The listing builds one solid part. Answer for the finished solid, in the listing's coordinates (mm). A direction names the side the tool comes from. Coordinates: 2 decimals unless noted, no trailing zeros. Order: outer loops, then holes, each group sorted by start corner. A loop starts at its lowest first (then second) coordinate and runs counter-clockwise, first axis right, second up. Notation, with made-up numbers: (57.5, 57) - (86.5, 57) arc R9 cw to (86.5, 72) - close; hole circle Ø1 at (80, 23.5). An arc over 180 degrees is marked (long way). Use one line per item in the form item = value. Start each with the question number.
Item 1: Section B-B, the plane z = 12.54 is taken. Write down the section's boundary in (x, y), and give its area (3 significant figures).
Item 2: The mould has two halves that part along Z. Classify faces 1 (the cylindrical face through (66.99, -12.727, 2.504)), 2 (the cylindrical face through (77.591, -2.576, 11.487)), 3 (the flat face through (83.4, -12.64, 12.44)): released by +Z, released by -Z, zero draft, split by the parting line, or undercut.
Item 3: Section D-D, the plane x = 42.5 is taken. Write down the section's boundary in (y, z), and give its area (3 significant figures).
Item 4: A tool of negligible diameter and unlimited length cuts with its end or side. For faces 4 (the flat face through (25.94, -12.64, 12.44)), 5 (the flat face through (71, -12, 5.08)), from which of +Z, -Z, +X, -X, +Y, -Y can it reach the whole face along a straight path? Write none if from no direction.
Item 5: Section A-A, the plane y = -10 is taken. Write down the section's boundary in (x, z).
Item 6: Consider line 1 along X through (y, z) = (-8.5, 13.5); line 2 along Z through (x, y) = (75, -2.5); line 3 along Y through (x, z) = (62.5, 14.5). Determine where each line is inside the solid, lowest interval first. Write a range as [from, to].
Item 7: Section C-C, the plane z = 16.5 is taken. Write down the section's boundary in (x, y).
Item 8: Each of these flat-tipped pins is pushed along its axis until it touches: pin 1 Ø10 at (x, y) = (39, -13) entering from +Z; pin 2 Ø8 at (y, z) = (-10, 17.5) entering from -X; pin 3 Ø12 at (x, z) = (74, 16) entering from -Y; pin 4 Ø1 at (x, z) = (60, 10.5) entering from -Y. Where does it stop, or does it pass through?
Autodesk Inventor part; units mm, degrees
ref_plane "YZ Plane" through (0, 0, 0) normal (1, 0, 0) x (0, 1, 0)
ref_plane "XZ Plane" through (0, 0, 0) normal (0, 1, 0) x (-1, 0, 0)
ref_plane "XY Plane" through (0, 0, 0) normal (0, 0, 1) x (1, 0, 0)
sketch "Sketch1" plane through (0, 0, 0) normal (0, 0, 1) x (1, 0, 0)
  line L0 (0, -1.25) -> (250, -1.25) construction
  line L1 (0, -1.25) -> (0, -6.4)
  line L2 (0, -6.4) -> (250, -6.4) construction
  line L3 (250, -1.25) -> (250, -6.4)
  line L4 (250, -18.75) -> (0, -18.75) construction
  line L5 (250, -13.6) -> (250, -18.75)
  line L6 (0, -13.6) -> (250, -13.6) construction
  line L7 (0, -13.6) -> (0, -18.75)
  line L8 (0, -20) -> (250, -20) construction
  line L9 (250, 0) -> (0, 0) construction
  line L10 (24.6484, -20) -> (84.6484, -20)
  line L11 (84.6484, -20) -> (84.6484, 0)
  line L12 (84.6484, 0) -> (24.6484, 0)
  line L13 (24.6484, 0) -> (24.6484, -20)
  line L14 (54.6484, -20) -> (54.6484, 0) construction
  circle A0 centre (67.3484, -10) radius 2.75
  circle A1 centre (41.9484, -10) radius 2.75
  line L15 (54.6484, -10) -> (41.9484, -10) construction
  line L16 (54.6484, -10) -> (67.3484, -10) construction
  point P0 (0, 0)
  dimension "d0" = 60
  dimension "d1" = 5.5
  dimension "d2" = 5.5
  dimension "d11" = 12.7
extrude "Extrusion1" add sketch "Sketch1" along normal blind 5.08
sketch "Sketch2" plane through (0, 0, 5.08) normal (0, 0, 1) x (1, 0, 0)
  line L0 (84.6484, 0) -> (24.6484, 0)
  line L1 (84.6484, -20) -> (84.6484, 0)
  line L2 (24.6484, 0) -> (84.6484, 0)
  line L3 (84.6484, 0) -> (84.6484, -5.08)
  line L4 (84.6484, -5.08) -> (24.6484, -5.08)
  line L5 (24.6484, -5.08) -> (24.6484, 0)
  point P0 (0, 0)
  dimension "d5" = 5.08
extrude "Extrusion2" add sketch "Sketch2" along normal blind 14.92
sketch "Sketch3" plane through (24.6484, -5.08, 5.08) normal (0, -1, 0) x (1, 0, 0)
  line L0 (0, -5.08) -> (0, 14.92)
  line L1 (0, 0) -> (60, 0)
  line L2 (0, 14.92) -> (0, 0)
  line L3 (60, -5.08) -> (60, 14.92)
  line L4 (19.1525, 952.0343) -> (19.1525, -47.9657) construction
  line L5 (19.1525, 952.0343) -> (14.0025, 952.0343)
  line L6 (14.0025, 952.0343) -> (14.0025, -47.9657) construction
  line L7 (19.1525, -47.9657) -> (14.0025, -47.9657)
  line L8 (1.6525, -47.9657) -> (1.6525, 952.0343) construction
  line L9 (6.8025, -47.9657) -> (1.6525, -47.9657)
  line L10 (6.8025, 952.0343) -> (6.8025, -47.9657) construction
  line L11 (6.8025, 952.0343) -> (1.6525, 952.0343)
  line L12 (0, 7.46) -> (1.6525, 7.46)
  line L13 (6.8025, 7.46) -> (14.0025, 7.46) construction
  line L14 (41.6525, -47.9657) -> (41.6525, 952.0343) construction
  line L15 (41.6525, -47.9657) -> (46.8025, -47.9657)
  line L16 (46.8025, -47.9657) -> (46.8025, 952.0343) construction
  line L17 (41.6525, 952.0343) -> (46.8025, 952.0343)
  line L18 (59.1525, 952.0343) -> (59.1525, -47.9657) construction
  line L19 (54.0025, 952.0343) -> (59.1525, 952.0343)
  line L20 (54.0025, -47.9657) -> (54.0025, 952.0343) construction
  line L21 (54.0025, -47.9657) -> (59.1525, -47.9657)
  line L22 (46.8025, 7.46) -> (54.0025, 7.46) construction
  line L23 (59.1525, 7.46) -> (60, 7.46)
  circle A0 centre (50.4025, 7.46) radius 2.75
  circle A1 centre (10.4025, 7.46) radius 2.75
  point P0 (-24.6484, -5.08)
  dimension "d8" = 5.5
extrude "Extrusion3" cut sketch "Sketch3" against normal blind 14.92
sketch "Sketch4" plane through (84.6484, -20, 0) normal (1, 0, 0) x (0, 0, -1)
  line L0 (-5.08, 0) -> (-5.08, 14.92)
  line L1 (-5.08, 14.92) -> (-20, 14.92)
  line L2 (-5.08, 0) -> (-20, 14.92)
  line L3 (-20, 14.92) -> (-5.08, 14.92)
  line L4 (-5.08, 14.92) -> (-5.08, 0)
  point P0 (0, 20)
extrude "Extrusion4" add sketch "Sketch4" against normal up to surface (60 mm away)
sketch "Sketch5" plane through (0, 0, 20) normal (0, 0, 1) x (1, 0, 0)
  line L0 (32.3009, 0) -> (37.8009, 0)
  line L1 (72.3009, 0) -> (77.8009, 0)
  circle A0 centre (41.9484, -10) radius 2.75
  circle A1 centre (67.3484, -10) radius 2.75
  line L2 (84.6484, 0) -> (24.6484, 0)
  line L3 (54.6484, 0) -> (54.6484, -20)
  line L4 (24.6484, -20) -> (84.6484, -20)
  line L5 (59.7284, -20) -> (49.5684, -20)
  line L6 (49.5684, -20) -> (49.5684, 0)
  line L7 (49.5684, 0) -> (59.7284, 0)
  line L8 (59.7284, 0) -> (59.7284, -20)
  line L9 (59.7284, -20) -> (49.5684, 0) construction
  line L10 (49.5684, -20) -> (59.7284, 0) construction
  line L11 (84.6484, -20) -> (82.1084, -20)
  line L12 (82.1084, -20) -> (82.1084, 0)
  line L13 (82.1084, 0) -> (84.6484, 0)
  line L14 (84.6484, 0) -> (84.6484, -20)
  line L15 (24.6484, -20) -> (27.1884, -20)
  line L16 (27.1884, -20) -> (27.1884, 0)
  line L17 (27.1884, 0) -> (24.6484, 0)
  line L18 (24.6484, 0) -> (24.6484, -20)
  line L19 (24.6484, -5.08) -> (84.6484, -5.08)
  line L20 (84.6484, 0) -> (24.6484, 0)
  line L21 (24.6484, 0) -> (24.6484, -5.08)
  line L22 (24.6484, -5.08) -> (84.6484, -5.08)
  line L23 (84.6484, -5.08) -> (84.6484, 0)
  line L24 (59.7284, -20) -> (82.1084, -20)
  line L25 (82.1084, -20) -> (82.1084, -5.08)
  line L26 (82.1084, -5.08) -> (59.7284, -5.08)
  line L27 (59.7284, -5.08) -> (59.7284, -20)
  line L28 (27.1884, -20) -> (49.5684, -20)
  line L29 (49.5684, -20) -> (49.5684, -5.08)
  line L30 (49.5684, -5.08) -> (27.1884, -5.08)
  line L31 (27.1884, -5.08) -> (27.1884, -20)
  point P0 (0, 0)
  point P1 (54.6484, -10)
  dimension "d14" = 2.54
  dimension "d15" = 2.54
  dimension "d16" = 10.16
extrude "Extrusion5" cut sketch "Sketch5" against normal blind 14.92 contours L19 L6 L4 L16 | L19 L12 L4 L8 | A0 | A1
properties part number "double90"
Response:
q1.outline = (24.65, -12.54) - (27.19, -12.54) - (27.19, -5.08) - (32.3, -5.08) - (32.3, 0) - (24.65, 0) - close; (37.8, -5.08) - (49.57, -5.08) - (49.57, -12.54) - (59.73, -12.54) - (59.73, -5.08) - (72.3, -5.08) - (72.3, 0) - (37.8, 0) - close; (77.8, -5.08) - (82.11, -5.08) - (82.11, -12.54) - (84.65, -12.54) - (84.65, 0) - (77.8, 0) - close
q1.area = 363 mm2
q2.face_1 = zero draft
q2.face_2 = undercut
q2.face_3 = released by +Z
q3.outline = (-20, 0) - (-12.69, 0) - (-12.69, 5.08) - (-20, 5.08) - close; (-7.31, 0) - (0, 0) - (0, 20) - (-5.08, 20) - (-5.08, 5.08) - (-7.31, 5.08) - close
q3.area = 150 mm2
q4.face_4 = +Z, +X, -X, -Y
q4.face_5 = +Z, -Y
q5.outline = (24.65, 0) - (39.2, 0) - (39.2, 5.08) - (27.19, 5.08) - (27.19, 15.08) - (24.65, 15.08) - close; (44.7, 0) - (64.6, 0) - (64.6, 5.08) - (59.73, 5.08) - (59.73, 15.08) - (49.57, 15.08) - (49.57, 5.08) - (44.7, 5.08) - close; (70.1, 0) - (84.65, 0) - (84.65, 15.08) - (82.11, 15.08) - (82.11, 5.08) - (70.1, 5.08) - close
q6.line_1 = [24.65, 27.19], [49.57, 59.73], [82.11, 84.65]
q6.line_2 = [0, 9.79], [15.29, 20]
q6.line_3 = [-5.08, 0]
q7.outline = (24.65, -8.58) - (27.19, -8.58) - (27.19, -5.08) - (49.57, -5.08) - (49.57, -8.58) - (59.73, -8.58) - (59.73, -5.08) - (82.11, -5.08) - (82.11, -8.58) - (84.65, -8.58) - (84.65, 0) - (24.65, 0) - close
q8.pin_1 = 5.08
q8.pin_2 = 24.65
q8.pin_3 = -5.08
q8.pin_4 = -15
